from build123d import *

# Parameters (mm, degrees)
F0_W        = 32
F0_H        = 3.5
F1_DEPTH    = 7.5
F2_DEPTH    = 7.5
F4_DEPTH    = 40
F5_T1_DEPTH = 30.4300979278


# Not quite as in the source:
# - a fillet or chamfer that OpenCascade refuses, or shapes differently, is made with other operations: its cross-section is extruded or revolved along the edge and cut away or added


with BuildPart() as f1:
    # F0 (on Right) → F1 (new body, symmetric)
    with BuildSketch(Plane.YZ):
        with Locations((0, -5.75)):
            Rectangle(F0_W, F0_H)
        Polygon((16, 0), (16, 4), (-16, 4), (-16, 0), (-16, -4), (16, -4), align=None)
        with Locations((0, 5.75)):
            Rectangle(F0_W, F0_H)
    extrude(amount=F1_DEPTH, both=True)

    # F0 (on Right) → F2 (join)
    with BuildSketch(Plane.YZ):
        with BuildLine():
            Line((-16, -4), (-16, 0))
            ThreePointArc((-16, 0), (-17.1715728753, -2.8284271247), (-20, -4))
            Line((-20, -4), (-16, -4))
        make_face()
        with BuildLine():
            ThreePointArc((-16, 0), (-17.1715728753, 2.8284271247), (-20, 4))
            Line((-20, 4), (-20, 1.75))
            ThreePointArc((-20, 1.75), (-18.7625631329, 1.2374368671), (-18.25, 0))
            ThreePointArc((-18.25, 0), (-18.7625631329, -1.2374368671), (-20, -1.75))
            Line((-20, -1.75), (-20, -4))
            ThreePointArc((-20, -4), (-17.1715728753, -2.8284271247), (-16, 0))
        make_face()
        with BuildLine():
            Line((-16, 0), (-16, 4))
            Line((-16, 4), (-20, 4))
            ThreePointArc((-20, 4), (-17.1715728753, 2.8284271247), (-16, 0))
        make_face()
        with BuildLine():
            Line((-20, 1.75), (-20, 4))
            ThreePointArc((-20, 4), (-24, 0), (-20, -4))
            Line((-20, -4), (-20, -1.75))
            ThreePointArc((-20, -1.75), (-21.75, 0), (-20, 1.75))
        make_face()
        with BuildLine():
            Line((20, 1.75), (20, 4))
            ThreePointArc((20, 4), (17.1715728753, 2.8284271247), (16, 0))
            ThreePointArc((16, 0), (17.1715728753, -2.8284271247), (20, -4))
            Line((20, -4), (20, -1.75))
            ThreePointArc((20, -1.75), (18.25, 0), (20, 1.75))
        make_face()
        with BuildLine():
            ThreePointArc((16, 0), (17.1715728753, 2.8284271247), (20, 4))
            Line((20, 4), (16, 4))
            Line((16, 4), (16, 0))
        make_face()
        with BuildLine():
            ThreePointArc((20, -4), (17.1715728753, -2.8284271247), (16, 0))
            Line((16, 0), (16, -4))
            Line((16, -4), (20, -4))
        make_face()
        with BuildLine():
            ThreePointArc((24, 0), (22.8284271247, 2.8284271247), (20, 4))
            Line((20, 4), (20, 1.75))
            ThreePointArc((20, 1.75), (21.2374368671, 1.2374368671), (21.75, 0))
            ThreePointArc((21.75, 0), (21.2374368671, -1.2374368671), (20, -1.75))
            Line((20, -1.75), (20, -4))
            ThreePointArc((20, -4), (22.8284271247, -2.8284271247), (24, 0))
        make_face()
    extrude(amount=F2_DEPTH)

    # F3 (on face) → F4 (cut)
    with BuildSketch(Plane.XZ.offset(16)):
        with BuildLine():
            ThreePointArc((1, 5.75), (0.7071067812, 6.4571067812), (0, 6.75))
            Line((0, 6.75), (0, 4.75))
            ThreePointArc((0, 4.75), (0.7071067812, 5.0428932188), (1, 5.75))
        make_face()
        with BuildLine():
            Line((0, 4.75), (0, 6.75))
            ThreePointArc((0, 6.75), (-1, 5.75), (0, 4.75))
        make_face()
        with BuildLine():
            ThreePointArc((1, -5.75), (0.7071067812, -5.0428932188), (0, -4.75))
            Line((0, -4.75), (0, -6.75))
            ThreePointArc((0, -6.75), (0.7071067812, -6.4571067812), (1, -5.75))
        make_face()
        with BuildLine():
            Line((0, -6.75), (0, -4.75))
            ThreePointArc((0, -4.75), (-1, -5.75), (0, -6.75))
        make_face()
    extrude(amount=-F4_DEPTH, mode=Mode.SUBTRACT)

    # F5: chamfer of 3 on 4 edges, made by hand

    # F5_s2 → F5_t1 (cut)
    with BuildSketch(Plane.YZ.offset(-15.2150489639)):
        Polygon((-13, 7.5), (-16, 4.5), (-16, 7.5), align=None)
        Polygon((-13, -7.5), (-16, -4.5), (-16, -7.5), align=None)
        Polygon((16, 4.5), (13, 7.5), (16, 7.5), align=None)
        Polygon((16, -4.5), (13, -7.5), (16, -7.5), align=None)
    extrude(amount=F5_T1_DEPTH, mode=Mode.SUBTRACT)


solid = f1.part
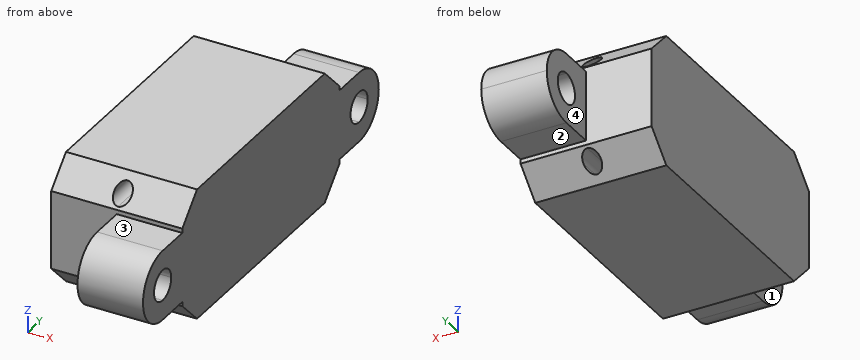
The model under review builds one solid part; all positions refer to its coordinate system, in mm. Face numbers are marked on the shaded views. A direction names the side the tool comes from. Give positions to 0.01 mm unless a question says otherwise; leave off trailing zeros. Order: outer loops, then holes, each group sorted by start corner. A loop starts at its lowest first (then second) coordinate and runs counter-clockwise, first axis right, second up. Notation, with made-up numbers: M 83.25,45.5 L 96.25,45.5 A6 cw 96.25,53.5 Z; hole C 16,58.5 d3. An arc over 180 degrees is marked long. Use one line per item in the form item = value. Start each with the question number.
Item 1: We need section C-C on x = -2.5. Give the boundary of the cut face in (y, z), plus the area to 3 significant figures.
Item 2: We need section B-B on y = 10. Give the boundary of the cut face in (x, z), plus the area to 3 significant figures.
Item 3: Insertion check: pin 1 Ø1.2 at (x, y) = (2.5, -17) entering from +Z; pin 2 Ø3 at (x, z) = (-0.5, 4.5) entering from -Y; pin 3 Ø4 at (y, z) = (19, 1.5) entering from -X. Each pin has a flat end and moves straight along its axis. Give the tip position at first contact, or say it passes through.
Item 4: To check wall thickness, follow line 1 along Y through (x, z) = (4.5, -0.5); line 2 along Y through (x, z) = (6.25, -1.5); line 3 along X through (y, z) = (18, 2.75). State the ranges of each line that lie inside material, in increasing order. Write a range as from..to.
Item 5: For the marked faces 1, 2, 3 and 4, list the 3-axis set-ups (+Z, -Z, +X, -X, +Y, -Y) from which the entire face can be reached by the end or side of a thin tool; tool diameter is ignored.
Item 6: We need section A-A on x = 2. Give the boundary of the cut face in (y, z).
Completed:
q1.outline = M -16,-4.5 L -13,-7.5 L 13,-7.5 L 16,-4.5 L 16,4.5 L 13,7.5 L -13,7.5 L -16,4.5 Z
q1.area = 462 mm²
q2.outline = M -7.5,-7.5 L 7.5,-7.5 L 7.5,7.5 L -7.5,7.5 Z; hole C 0,-5.75 d2; hole C 0,5.75 d2
q2.area = 219 mm²
q3.pin_1 = 4
q3.pin_2 = -22.55
q3.pin_3 = 0
q4.line_1 = -23.97..-21.68, -18.32..18.32, 21.68..23.97
q4.line_2 = -23.71..-20.9, -19.1..19.1, 20.9..23.71
q4.line_3 = 0..7.5
q5.face_1 = +Z, -Z, -X, -Y
q5.face_2 = -Z, +X, -X, +Y
q5.face_3 = +Z, +X, -X, -Y
q5.face_4 = +Z, -Z, -X, +Y
q6.outline = M -20,-4 L -16,-4 L -16,-4.5 L -13,-7.5 L 13,-7.5 L 16,-4.5 L 16,-4 L 20,-4 A4 ccw 20,4 L 16,4 L 16,4.5 L 13,7.5 L -13,7.5 L -16,4.5 L -16,4 L -20,4 A4 ccw Z; hole C -20,0 d3.5; hole C 20,0 d3.5
